Geometry check sheet. Reference: drawing and pictorial views, mm from the part's lowest x, y, z. Coordinates: 2 decimals unless noted, no trailing zeros. Write each loop counter-clockwise with the first axis right and the second up, starting at its lowest first coordinate (ties: lowest second). Pieces come first, ordered by that corner, then holes. Notation, with made-up numbers: (88, 36) -> (93, 36) arc R13 ccw to (93, 42) -> close; hole circle Ø3 at (52, -22). An arc over 180 degrees is marked (long way). Put each result on its own line as item: value.
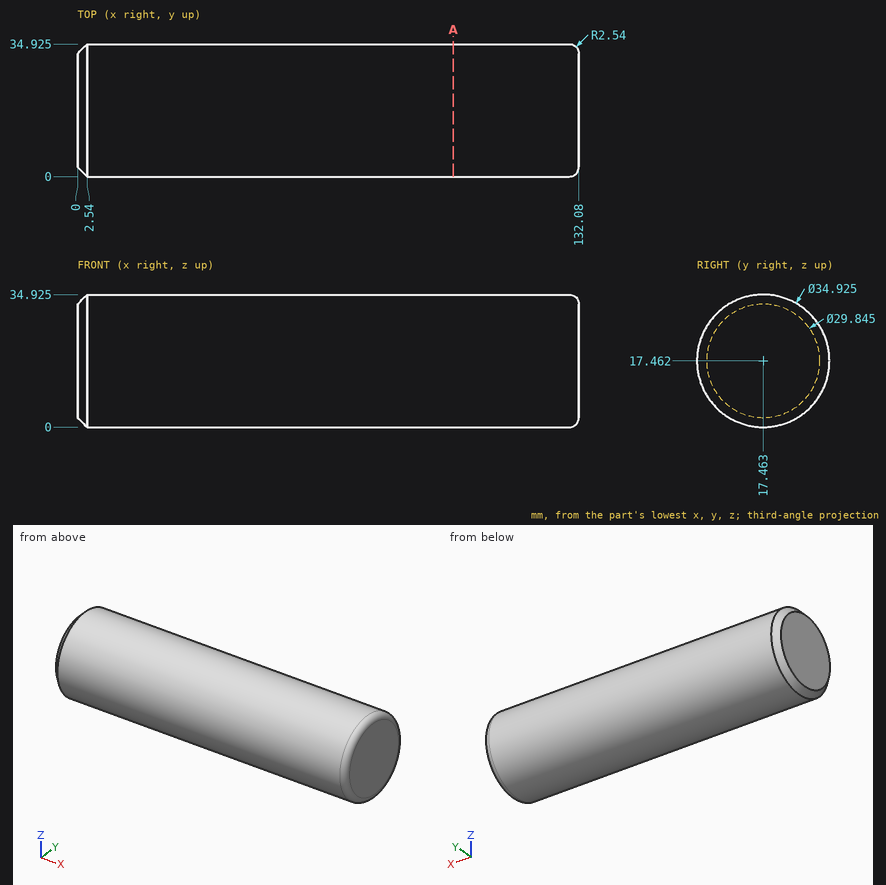
Q1. Cross-section at A-A (x = 99). Record the cut outline in (y, z) (1 decimal), plus the area to 3 significant figures.
Recorded:
outline: circle Ø34.9 at (17.5, 17.5)
area: 958 mm2
Q2. Material ranges on line 1 along Z through (x, y) = (59.5, 16.5); line 2 along Z through (x, y) = (113.5, 8) (1 decimal); line 3 along X through (y, z) = (4, 24) (1 decimal), recorded low to high.
Recorded:
line 1: z = 0.03 to 34.9
line 2: z = 2.8 to 32.1
line 3: x = 0 to 132.1
Q3. Depth check by flat-ended pin: P1, Ø6, axis at x = 88.5, z = 6.5, coming from the -Y side; P2, Ø1.5, axis at x = 44.5, z = 13.5, coming from the +Y side; P3, Ø10, axis at x = 51.5, y = 4, coming from the -Z side. Enter the tip coordinate at first touch or a pass-through.
Recorded:
P1: stops at y = 1.92
P2: stops at y = 34.63
P3: stops at z = 2.19
